Work out the finished part from the listing and answer in its coordinate system (mm). A direction names the side the tool comes from. Give positions to 0.01 mm unless a question says otherwise; leave off trailing zeros. Loops run counter-clockwise (first coordinate to the right, second up) from the corner with the lowest first, then second, coordinate; pieces in that order, holes last. Notation, with made-up numbers: (74, 22) -> (133, 22) arc R27 ccw to (133, 40) -> close; hole circle Ø1 at (2, 61). An arc over 180 degrees is marked (long way). Answer as CSV lines item,"result". Start each with the question number.
1. Find section B-B, the plane z = 62. Give the vertices of the cut face in (x, y).
2. Find section D-D, the plane y = 47. Give the vertices of the cut face in (x, z).
3. Find the intervals of material crossed by line 1 along X through (y, z) = (38.1, 102.75); line 2 along X through (y, z) = (12.7, 102.75); line 3 along Z through (x, y) = (-104, 58), in increasing order.
4. A tool of negligible diameter and unlimited length cuts with its end or side. For faces 4 (the face through (-147.904, 8.26, 102.835)), 5 (the face through (-96, 38, 98.006)), 6 (the face through (-115.29, 61.79, 102.83)), 7 (the face through (-118, 46, 63.081)), 8 (the face through (-118, 69.85, 103)), from which of +Z, -Z, +X, -X, +Y, -Y can it reach the whole face along a straight path? Write none if from no direction.
5. Find section A-A, the plane y = 38.1. Give the vertices of the cut face in (x, z).
6. Flat-ended cylindrical pins translate along their axes: pin 1 Ø2 at (x, y) = (-109.5, 30) entering from -Z; pin 2 Ø5.5 at (x, y) = (-92.56, 63.5) entering from +Z; pin 3 Ø7.5 at (x, z) = (-130, 103) entering from +Y. Find the tip coordinate at first contact, or state that the pin passes through.
7. Determine the mould class of faces 1 (the face through (-140.217, 13.113, 102.835)), 2 (the face through (-88.026, 67.94, 102.835)), 3 (the face through (-149.715, 38, 103)) for opening direction Y: +Y half, -Y half, draft (parallel to the pull), parting line (faces both ways), or undercut.
8. Find section C-C, the plane x = -141.5. Give the vertices of the cut face in (y, z), and give its area (3 significant figures).
Solid Edge part; units mm, degrees
sketch "Sketch1" plane through (0, 0, 0) normal (0, -1, 0) x (1, 0, 0)
  line L0 (-149.7149, 69.4306) -> (-86.2149, 69.4306)
  line L1 (-86.2149, 69.4306) -> (-86.2149, 56.7306)
  line L2 (-86.2149, 56.7306) -> (-98.9149, 56.7306)
  line L3 (-92.5649, 63.0806) -> (-98.9149, 56.7306)
  line L4 (-143.3649, 63.0806) -> (-92.5649, 63.0806)
  line L5 (-143.3649, 63.0806) -> (-137.0149, 56.7306)
  line L6 (-137.0149, 56.7306) -> (-149.7149, 56.7306)
  line L7 (-149.7149, 56.7306) -> (-149.7149, 69.4306)
extrude "Protrusion1" add sketch "Sketch1" against normal blind 76.2
sketch "Sketch2" plane through (-117.9649, 38.1, 69.4306) normal (0, 0, 1) x (1, 0, 0)
  line L0 (31.75, -31.75) -> (-31.75, -31.75)
  line L1 (-31.75, -31.75) -> (-31.75, 31.75)
  line L2 (-31.75, 31.75) -> (31.75, 31.75)
  line L3 (31.75, 31.75) -> (31.75, -31.75)
extrude "ExtrudedProtrusion_2" add sketch "Sketch2" along normal blind 38.1
sketch "Sketch3" plane through (-117.9649, 6.35, 88.4806) normal (0, -1, 0) x (1, 0, 0)
  line L0 (-31.75, -9.525) -> (-19.05, -9.525)
  line L1 (-19.05, 9.525) -> (-19.05, -9.525)
  line L2 (-31.75, 9.525) -> (-19.05, 9.525)
extrude "Cutout1" cut sketch "Sketch3" against normal through all material side at (-143.3649, 6.35, 79.0056)
sketch "Sketch4" plane through (-117.9649, 6.35, 88.4806) normal (0, -1, 0) x (1, 0, 0)
  line L0 (19.05, -9.525) -> (31.75, -9.525)
  line L1 (19.05, 9.525) -> (19.05, -9.525)
  line L2 (31.75, 9.525) -> (19.05, 9.525)
extrude "Cutout2" cut sketch "Sketch4" against normal through all material side at (-92.5649, 6.35, 79.0056)
sketch "Sketch5" plane through (-98.9149, 38.1, 88.4806) normal (1, 0, 0) x (0, 0, -1)
  line L0 (-9.525, 19.05) -> (9.525, 19.05)
  line L1 (9.525, 19.05) -> (9.525, 31.75)
  line L2 (9.525, 31.75) -> (-9.525, 31.75)
  line L3 (-9.525, 31.75) -> (-9.525, 19.05)
  line L4 (-9.525, -19.05) -> (9.525, -19.05)
  line L5 (9.525, -19.05) -> (9.525, -31.75)
  line L6 (9.525, -31.75) -> (-9.525, -31.75)
  line L7 (-9.525, -31.75) -> (-9.525, -19.05)
extrude "Cutout3" cut sketch "Sketch5" against normal through all
hole "Hole_2" at (-92.5649, 63.5, 107.5306) direction (0, 0, -1) diameter 6.35 end up to next
hole "Hole_11" at (-117.9649, 63.5, 107.5306) direction (0, 0, -1) diameter 6.35 end up to next
hole "Hole1" at (-143.3649, 63.5, 107.5306) direction (0, 0, -1) diameter 6.35 end up to next
hole "Hole2" at (-143.3649, 38.1, 107.5306) direction (0, 0, -1) diameter 6.35 end up to next
hole "Hole3" at (-143.3649, 12.7, 107.5306) direction (0, 0, -1) diameter 6.35 end up to next
hole "Hole4" at (-117.9649, 12.7, 107.5306) direction (0, 0, -1) diameter 6.35 end up to next
hole "Hole5" at (-92.5649, 12.7, 107.5306) direction (0, 0, -1) diameter 6.35 end up to next
hole "Hole6" at (-92.5649, 38.1, 107.5306) direction (0, 0, -1) diameter 6.35 end up to next
hole "Hole_18" at (-117.9649, 38.1, 107.5306) direction (0, 0, -1) diameter 12.7 end up to next
fillet "Round_1" radius 6.35 8 edges at (-149.7149, 69.85, 74.1931) (-149.7149, 6.35, 74.1931) (-86.2149, 69.85, 74.1931) (-86.2149, 6.35, 74.1931) (-149.7149, 6.35, 102.7681) (-149.7149, 69.85, 102.7681) (-86.2149, 6.35, 102.7681) (-86.2149, 69.85, 102.7681)
Resolved:
1,outline,"(-149.71, 0) -> (-142.28, 0) -> (-142.28, 76.2) -> (-149.71, 76.2) -> close; (-93.65, 0) -> (-86.21, 0) -> (-86.21, 76.2) -> (-93.65, 76.2) -> close"
2,outline,"(-149.71, 56.73) -> (-137.01, 56.73) -> (-143.36, 63.08) -> (-92.56, 63.08) -> (-98.91, 56.73) -> (-86.21, 56.73) -> (-86.21, 78.96) -> (-98.91, 78.96) -> (-98.91, 98.01) -> (-86.21, 98.01) -> (-86.21, 107.53) -> (-149.71, 107.53) -> (-149.71, 98.01) -> (-137.01, 98.01) -> (-137.01, 78.96) -> (-149.71, 78.96) -> close"
3,line 1,"x = -149.71 to -146.54, -140.19 to -124.31, -111.61 to -95.74, -89.39 to -86.21"
3,line 2,"x = -149.71 to -146.54, -140.19 to -121.14, -114.79 to -95.74, -89.39 to -86.21"
3,line 3,"z = 63.08 to 78.96, 98.01 to 107.53"
4,face 4,"+Z, -X, -Y"
4,face 5,"none"
4,face 6,"+Z"
4,face 7,"+Y, -Y"
4,face 8,"+Z, +X, -X, +Y"
5,outline,"(-149.71, 56.73) -> (-137.01, 56.73) -> (-143.36, 63.08) -> (-124.31, 63.08) -> (-124.31, 107.53) -> (-140.19, 107.53) -> (-140.19, 98.01) -> (-137.01, 98.01) -> (-137.01, 78.96) -> (-149.71, 78.96) -> close; (-149.71, 98.01) -> (-146.54, 98.01) -> (-146.54, 107.53) -> (-149.71, 107.53) -> close; (-111.61, 63.08) -> (-92.56, 63.08) -> (-98.91, 56.73) -> (-86.21, 56.73) -> (-86.21, 78.96) -> (-98.91, 78.96) -> (-98.91, 98.01) -> (-95.74, 98.01) -> (-95.74, 107.53) -> (-111.61, 107.53) -> close; (-89.39, 98.01) -> (-86.21, 98.01) -> (-86.21, 107.53) -> (-89.39, 107.53) -> close"
6,pin 1,"stops at z = 63.08"
6,pin 2,"stops at z = 78.96"
6,pin 3,"stops at y = 69.85"
7,face 1,"undercut"
7,face 2,"+Y half"
7,face 3,"draft"
8,outline,"(0, 56.73) -> (76.2, 56.73) -> (76.2, 61.22) -> (0, 61.22) -> close; (0, 63.08) -> (76.2, 63.08) -> (76.2, 69.43) -> (69.85, 69.43) -> (69.85, 78.96) -> (6.35, 78.96) -> (6.35, 69.43) -> (0, 69.43) -> close; (6.35, 98.01) -> (10.13, 98.01) -> (10.13, 107.53) -> (6.35, 107.53) -> close; (15.27, 98.01) -> (35.53, 98.01) -> (35.53, 107.53) -> (15.27, 107.53) -> close; (40.67, 98.01) -> (60.93, 98.01) -> (60.93, 107.53) -> (40.67, 107.53) -> close; (66.07, 98.01) -> (69.85, 98.01) -> (69.85, 107.53) -> (66.07, 107.53) -> close"
8,area,"1,890 mm^2"
